Geometry check sheet. Reference: the model listing, model coordinates, mm. Coordinates: 2 decimals unless noted, no trailing zeros. Write each loop counter-clockwise with the first axis right and the second up, starting at its lowest first coordinate (ties: lowest second). Pieces come first, ordered by that corner, then holes. Notation, with made-up numbers: (12.5, -31) -> (68.5, -31) arc R28 cw to (68.5, 3) -> close; hole circle Ø11 at (60.5, 17). An arc over 180 degrees is marked (long way). Answer in a Markdown table with one row per item. Add a question column.
Q1. Release check for a two-part mould opening along X. For faces 1 (the face through (-8.992, 27.055, -1.655)), 2 (the face through (-17.239, 40.245, -1.655)), 3 (the face through (0, 1, -3.264)), 4 (the face through (17.14, 40.344, -1.655)) record: pulls with the +X half, pulls with the -X half, needs draft (parallel to the pull), parting line crosses it, or undercut.
Q2. Section check B-B, the plane z = -2.3. Record the boundary of the cut face in (x, y) (3 decimals).
Q3. Thickness scan on line 1 (X direction, y = 29.5, z = -1.15); line 2 (Y direction, x = -8, z = -2.9); line 3 (Y direction, x = -7.5, z = -0.95). Record the ranges inside material, lowest first.
Q4. Gauge pin test, flat ends, axial feed: P1, Ø1, axis at x = 15, z = -2, coming from the +Y side; P2, Ø3, axis at x = 9.52, y = 29.45, coming from the -Z side. Record the tip position at first contact, or that the pin passes through.
Q5. Section check A-A, the plane x = 11. Record the boundary of the cut face in (y, z).
```python
from build123d import *

# Parameters (mm, degrees)
SKETCH1_W                    = 38.1
SKETCH1_H                    = 84.30895
BASE_FLANGE1_DEPTH           = 3.2639
F_10_0_1935_DIAMETER_HOLE1_D = 4.9149
FILLET1_R                    = 6.35


# Sheet-metal steps are written as plain solids
with BuildPart() as part:
    # Sketch1 → Base-Flange1 (new body)
    with BuildSketch(Plane.XY):
        Rectangle(SKETCH1_W, SKETCH1_H)
    extrude(amount=-BASE_FLANGE1_DEPTH)

    # #10 (0.1935) Diameter Hole1 (through all)
    with Locations(Plane.XY):
        with Locations((-9.525, 29.454475), (9.525, 29.454475)):
            Hole(F_10_0_1935_DIAMETER_HOLE1_D / 2)

    # Fillet1
    fillet1_edges = [part.edges().sort_by_distance(p)[0] for p in [
        (-19.05, 42.154475, -1.63195),
        (19.05, 42.154475, -1.63195),
    ]]
    fillet(fillet1_edges, radius=FILLET1_R)


solid = part.part
```
Calculated:
| question | item | result |
|---|---|---|
| 1 | face 1 | undercut |
| 1 | face 2 | pulls with the -X half |
| 1 | face 3 | needs draft |
| 1 | face 4 | pulls with the +X half |
| 2 | outline | (-19.05, -42.154) -> (19.05, -42.154) -> (19.05, 35.804) arc R6.35 ccw to (12.7, 42.154) -> (-12.7, 42.154) arc R6.35 ccw to (-19.05, 35.804) -> close; hole circle Ø4.915 at (-9.525, 29.454); hole circle Ø4.915 at (9.525, 29.454) |
| 3 | line 1 | x = -19.05 to -11.98, -7.07 to 7.07, 11.98 to 19.05 |
| 3 | line 2 | y = -42.15 to 27.53, 31.38 to 42.15 |
| 3 | line 3 | y = -42.15 to 28.06, 30.85 to 42.15 |
| 4 | P1 | stops at y = 41.89 |
| 4 | P2 | passes through |
| 5 | outline | (-42.15, -3.26) -> (27.49, -3.26) -> (27.49, 0) -> (-42.15, 0) -> close; (31.42, -3.26) -> (42.15, -3.26) -> (42.15, 0) -> (31.42, 0) -> close |
